Geometry check sheet. Reference: drawing and pictorial views, mm from the part's lowest x, y, z. A direction names the side the tool comes from. Give positions to 0.01 mm unless a question says otherwise; leave off trailing zeros. Order: outer loops, then holes, each group sorted by start corner. A loop starts at its lowest first (then second) coordinate and runs counter-clockwise, first axis right, second up.
Item 1: Sectioned sample at A-A on x = 26.5. Record the boundary of the cut face in (y, z), and give its area (3 significant figures).
Item 2: Release check for a two-part mould opening along Z. For the marked faces 6, 7, 8 and 9 record: released by +Z, released by -Z, zero draft, split by the parting line, or undercut.
Item 3: Sectioned sample at D-D on z = 85. Record the boundary of the cut face in (x, y), and give its area (3 significant figures).
Item 4: Sectioned sample at C-C on x = 9. Record the boundary of the cut face in (y, z).
Item 5: Material ranges on line 1 along Z through (x, y) = (13, 16.25); line 2 along X through (y, z) = (11.25, 139.5); line 3 along X through (y, z) = (4, 72.5), recorded low to high.
Item 6: Sectioned sample at B-B on y = 20.5. Record the boundary of the cut face in (x, z), and give its area (3 significant figures).
Item 7: Access from +Z, -Z, +X, -X, +Y, -Y to the whole of each face (thin tool, end or side, straight path). Record for the marked faces 1, 2, 3, 4 and 5.
Item 8: Gauge pin test, flat ends, axial feed: P1, Ø9.5, axis at y = 18.5, z = 73, coming from the -X side; P2, Ø1.5, axis at x = 28.5, y = 8.5, coming from the +Z side; P3, Ø12.5, axis at y = 10, z = 119.5, coming from the -X side. Record the tip position at first contact, or that the pin passes through.
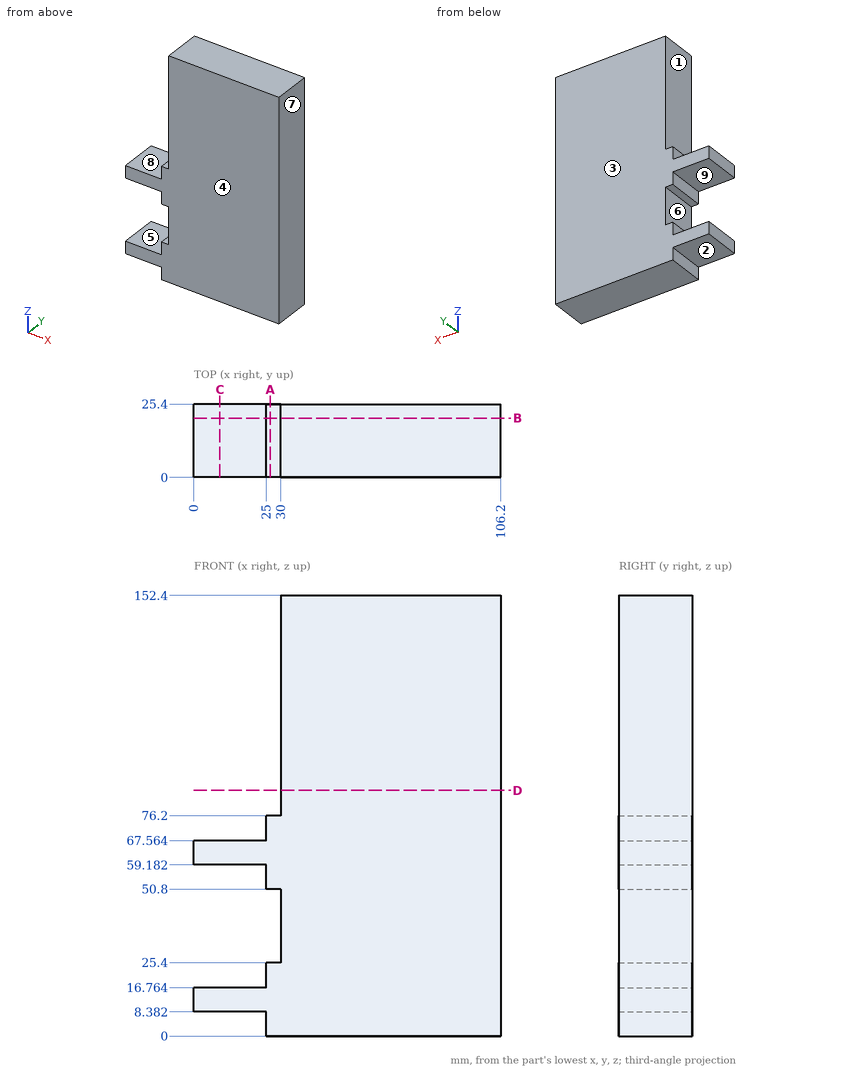
Report:
1. outline: (0, 0) - (25.4, 0) - (25.4, 25.4) - (0, 25.4) - close; (0, 50.8) - (25.4, 50.8) - (25.4, 76.2) - (0, 76.2) - close
1. area: 1,290 mm2
2. face 6: undercut
2. face 7: zero draft
2. face 8: released by +Z
2. face 9: undercut
3. outline: (30, 0) - (106.2, 0) - (106.2, 25.4) - (30, 25.4) - close
3. area: 1,940 mm2
4. outline: (0, 8.38) - (25.4, 8.38) - (25.4, 16.76) - (0, 16.76) - close; (0, 59.18) - (25.4, 59.18) - (25.4, 67.56) - (0, 67.56) - close
5. line 1: z = 8.38 to 16.76, 59.18 to 67.56
5. line 2: x = 30 to 106.2
5. line 3: x = 25 to 106.2
6. outline: (0, 8.38) - (25, 8.38) - (25, 0) - (106.2, 0) - (106.2, 152.4) - (30, 152.4) - (30, 76.2) - (25, 76.2) - (25, 67.56) - (0, 67.56) - (0, 59.18) - (25, 59.18) - (25, 50.8) - (30, 50.8) - (30, 25.4) - (25, 25.4) - (25, 16.76) - (0, 16.76) - close
6. area: 12,300 mm2
7. face 1: +Z, -X, +Y, -Y
7. face 2: -Z, -X, +Y, -Y
7. face 3: +Z, -Z, +X, -X, +Y
7. face 4: +Z, -Z, +X, -X, -Y
7. face 5: -X, +Y, -Y
8. P1: stops at x = 25
8. P2: stops at z = 76.2
8. P3: stops at x = 30
